from build123d import *

# Parameters (mm, degrees)
SKETCH1_R           = 1.905
BOSS_EXTRUDE1_DEPTH = 9.525
FILLET1_R           = 2.54
CHAMFER1_SIZE       = 0.635


with BuildPart() as part:
    # Sketch1 → Boss-Extrude1 (new body, symmetric)
    with BuildSketch(Plane(origin=(0, 0, 0), x_dir=(1, 0, 0), z_dir=(0, 1, 0))):
        with BuildLine():
            ThreePointArc((3.572376077, -3.149529395), (3.298614691, 0), (3.572376077, 3.149529395))
            ThreePointArc((3.572376077, 3.149529395), (-4.7625, 0), (3.572376077, -3.149529395))
        make_face()
        Circle(SKETCH1_R, mode=Mode.SUBTRACT)
    extrude(amount=BOSS_EXTRUDE1_DEPTH, both=True)

    # Fillet1
    fillet1_edges = [part.edges().sort_by_distance(p)[0] for p in [
        (3.572376077, 0, -3.149529395),
        (3.572376077, 0, 3.149529395),
    ]]
    fillet(fillet1_edges, radius=FILLET1_R)

    # Chamfer1
    chamfer1_edges = [part.edges().sort_by_distance(p)[0] for p in [
        (-4.7625, -9.525, 0),
        (-4.7625, 9.525, 0),
        (3.298614691, -9.525, 0),
        (3.041807621, -9.525, 3.349691374),
        (3.041807621, -9.525, -3.349691374),
        (3.298614691, 9.525, 0),
        (3.041807621, 9.525, 3.349691374),
        (3.041807621, 9.525, -3.349691374),
        (-1.905, -9.525, 0),
        (-1.905, 9.525, 0),
    ]]
    chamfer(chamfer1_edges, length=CHAMFER1_SIZE)


solid = part.part
The model under review builds one solid part; all positions refer to its coordinate system, in mm. Coordinates: 2 decimals unless noted, no trailing zeros. Loops run counter-clockwise (first coordinate to the right, second up) from the corner with the lowest first, then second, coordinate; pieces in that order, holes last. Notation, with made-up numbers: M 28.5,74 L 37.5,74 A25 cw 37.5,92 Z; hole C -12,-33.75 d2. An arc over 180 degrees is marked long. Put each result on its own line as item: value. Start each with the question number.
Q1. Clearance check with flat-ended pins moving along their axes: pin 1 (1 mm diameter, centred on y = 0, z = -2.5, fed in from +X); pin 2 (1 mm diameter, centred on x = -3.5, y = -3.5, fed in from -Z); pin 3 (1.5 mm diameter, centred on x = -2.5, y = 4.5, fed in from +Z). State where each tip first meets the part, or that it passes through.
Q2. Add section A-A (x = 0). Write out the cut boundary in (y, z) (1 decimal), and give its area (3 significant figures).
Q3. The part is to be moulded in two halves that separate along X. For faces 1 (the cylindrical face through (-4.76, 0.12, -0.13)), 2 (the cylindrical face through (-0.41, -0.12, 1.86)), 3 (the cylindrical face through (3.3, 0.1, 0)), 4 (the flat face through (-3, 9.525, 0)), say which applies: +X half, -X half, draft (parallel to the pull), parting line (faces both ways), or undercut.
Q4. Wall thickness on line 1 (Z direction, x = 0, y = 5) (1 decimal); line 2 (Z direction, x = -1.5, y = 0); line 3 (X direction, y = -8.5, z = 0.5): over which ranges is each line inside the solid? List them lowest first.
Answers:
1. pin 1: stops at x = 3.4
1. pin 2: stops at z = -3.7
1. pin 3: stops at z = 4.43
2. outline: M -9.5,-4.1 L -8.9,-4.8 L 8.9,-4.8 L 9.5,-4.1 L 9.5,-2.5 L 8.9,-1.9 L -8.9,-1.9 L -9.5,-2.5 Z; M -9.5,2.5 L -8.9,1.9 L 8.9,1.9 L 9.5,2.5 L 9.5,4.1 L 8.9,4.8 L -8.9,4.8 L -9.5,4.1 Z
2. area: 107 mm^2
3. face 1: parting line
3. face 2: undercut
3. face 3: +X half
3. face 4: draft
4. line 1: z = -4.8 to -1.9, 1.9 to 4.8
4. line 2: z = -4.52 to -1.17, 1.17 to 4.52
4. line 3: x = -4.74 to -1.84, 1.84 to 3.31
